Geometry check sheet. Reference: the model listing, model coordinates, mm. Coordinates: 2 decimals unless noted, no trailing zeros. Loops run counter-clockwise (first coordinate to the right, second up) from the corner with the lowest first, then second, coordinate; pieces in that order, holes last.
from build123d import *

# Parameters (mm, degrees)
F4_D     = 5
F4_DEPTH = 5
F4_TIP   = 1.5021515476


with BuildPart() as f1:
    # F0 (on Front) → F1 (revolve)
    with BuildSketch(Plane.XZ):
        with BuildLine():
            Line((209, 9.5), (2, 9.5))
            ThreePointArc((2, 9.5), (0.5054206912, 4.8541219597), (0, 0))
            Line((0, 0), (211, 0))
            ThreePointArc((211, 0), (210.4945793088, 4.8541219597), (209, 9.5))
        make_face()
    revolve(axis=Axis((104.3779142201, 0, 0), (1, 0, 0)))

    # F4
    with Locations(Plane.XY.offset(9.5)):
        with Locations((50, 0)):
            Hole(F4_D / 2, depth=F4_DEPTH)
            with Locations((0, 0, -(F4_DEPTH + F4_TIP / 2))):  # 118° drill point
                Cone(0, F4_D / 2, F4_TIP, mode=Mode.SUBTRACT)

    # F5 (on Front) → F6 (revolve, cut)
    with BuildSketch(Plane.XZ):
        Polygon((184.5, 11.5), (179, 11.5), (179, 6), align=None)
    revolve(axis=Axis((179, 0, -0.0294297934), (0, 0, -1)), mode=Mode.SUBTRACT)


solid = f1.part
1) Section check B-B on z = -7.5. Record the cut outline in (x, y).
Data:
outline: (2, -5.83) - (209, -5.83) arc R22.34 ccw to (209, 5.83) - (2, 5.83) arc R22.34 ccw to start
2) Material ranges on probe 1 along X at (y, z) = (0, 8.1); probe 2 along Z at (x, y) = (163, 0.5); probe 3 along Y at (x, z) = (50, 6.8), recorded low to high.
Data:
probe 1: x = 1.44 to 47.5, 52.5 to 176.9, 181.1 to 209.56
probe 2: z = -9.49 to 9.49
probe 3: y = -6.63 to -2.5, 2.5 to 6.63
3) Section check A-A on x = 103. Record the cut outline in (y, z), and give its area (3 significant figures).
Data:
outline: circle Ø19 at (0, 0)
area: 284 mm2
4) Mould release check, pull along Y, two halves, no side actions. Record for faces 1 (the conical face through (50, 0, 3)), 2 (the conical face through (180, 0, 7)), 3 (the cylindrical face through (104.05, 8.43, 4.38)): +Y half, -Y half, draft (parallel to the pull), parting line (faces both ways), or undercut.
Data:
face 1: undercut
face 2: undercut
face 3: parting line
5) Depth check by flat-ended pin: pin 1 (6 mm diameter, centred on x = 38.5, y = 5.5, fed in from -Z); pin 2 (2 mm diameter, centred on y = -1.5, z = 5, fed in from +X); pin 3 (10 mm diameter, centred on x = 147.5, z = -6.5, fed in from +Y). Enter the tip coordinate at first touch or a pass-through.
Data:
pin 1: stops at z = -9.17
pin 2: stops at x = 210.62
pin 3: stops at y = 9.38
